Autodesk Inventor part; units mm, degrees
ref_plane "YZ Plane" through (0, 0, 0) normal (1, 0, 0) x (0, 1, 0)
ref_plane "XZ Plane" through (0, 0, 0) normal (0, 1, 0) x (-1, 0, 0)
ref_plane "XY Plane" through (0, 0, 0) normal (0, 0, 1) x (1, 0, 0)
sketch "Sketch1" plane through (0, 0, 0) normal (0, 0, 1) x (1, 0, 0)
  line L0 (0, 0) -> (12.7, 0)
  line L1 (12.7, 0) -> (12.7, -12.7)
  line L2 (0, 0.762) -> (12.3844, 0.762)
  line L3 (13.462, -0.3156) -> (13.462, -12.7)
  line L4 (0, 0.762) -> (0, 0)
  line L5 (12.7, -12.7) -> (13.462, -12.7)
  arc A0 (13.462, -0.3156) -> (12.3844, 0.762) centre (13.462, 0.762) ccw
  dimension "d0" = 12.7
  dimension "d1" = 12.7
  dimension "d2" = 0.762
extrude "Extrusion1" add sketch "Sketch1" along normal blind 25.4
properties part number "Hinge_Rear" material "Brass, Soft Yellow"
Read the model definition and answer for the solid it produces. Units are mm, in the model's axes. A direction names the side the tool comes from. Coordinates: 2 decimals unless noted, no trailing zeros. Order: outer loops, then holes, each group sorted by start corner. A loop starts at its lowest first (then second) coordinate and runs counter-clockwise, first axis right, second up. Notation, with made-up numbers: (73, 51) - (127, 51) arc R13 ccw to (127, 67) - close; hole circle Ø7 at (69, 75.25). An arc over 180 degrees is marked (long way). Use one line per item in the form item = value.
(1) Given pin 1 Ø5 at (y, z) = (-7.5, 18.5) entering from -X; pin 2 Ø8 at (y, z) = (-0.5, 10) entering from -X; pin 3 Ø4 at (x, z) = (5, 15) entering from -Y; pin 4 Ø2 at (x, z) = (9.5, 8) entering from +Y, each flat-ended and moving along its own axis, determine where each tip first touches the part or whether it passes through.
Computed values:
pin_1 = 12.7
pin_2 = 0
pin_3 = 0
pin_4 = 0.76
(2) Which of the six approach directions +Z, -Z, +X, -X, +Y, -Y give full straight-line access (tool end or side, diameter ignored) to faces 1 (the face through (6, 0.762, 13)), 2 (the face through (12.7, -6, 13)), 3 (the face through (13.462, -6, 13))?
Computed values:
face_1 = +Z, -Z, -X, +Y
face_2 = +Z, -Z, -X, -Y
face_3 = +Z, -Z, +X, -Y
(3) Section A-A, the plane z = 9.5 is taken. Give the vertices of the cut face in (x, y), then the cut area to 3 significant figures.
Computed values:
outline = (0, 0) - (12.7, 0) - (12.7, -12.7) - (13.46, -12.7) - (13.46, -0.32) arc R1.08 ccw (long way) to (12.38, 0.76) - (0, 0.76) - close
area = 22.7 mm²
(4) Straight lines are drawn through the part: L1, parallel to X at y = -8, z = 18.5; L2, parallel to Y at x = 8.5, z = 9.75; L3, parallel to Y at x = 13, z = 2. For each, find the intervals that lie inside material, in ascending order.
Computed values:
L1 = 12.7 to 13.46
L2 = 0 to 0.76
L3 = -12.7 to 1.74
(5) Section C-C, the plane y = -6 is taken. Give the vertices of the cut face in (x, z).
Computed values:
outline = (12.7, 0) - (13.46, 0) - (13.46, 25.4) - (12.7, 25.4) - close
(6) Section B-B, the plane x = 12 is taken. Give the vertices of the cut face in (y, z), then the cut area to 3 significant figures.
Computed values:
outline = (0, 0) - (0.76, 0) - (0.76, 25.4) - (0, 25.4) - close
area = 19.4 mm²
